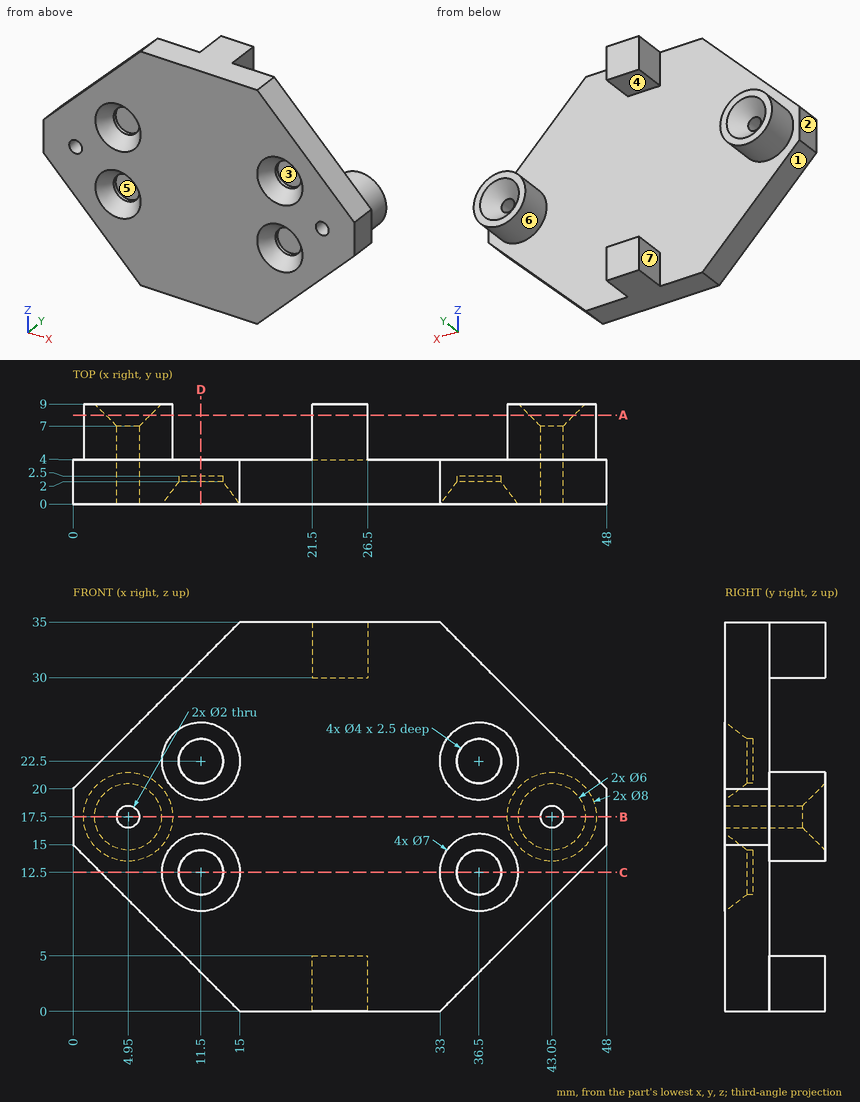
Input: dimensioned drawing with shaded views. Units: mm. Origin: part minimum x, y, z. A direction names the side the tool comes from. Coordinates: 2 decimals unless noted, no trailing zeros. Order: outer loops, then holes, each group sorted by start corner. A loop starts at its lowest first (then second) coordinate and runs counter-clockwise, first axis right, second up. Notation, with made-up numbers: (24.5, -2) -> (73.5, -2) arc R19 cw to (73.5, 19) -> close; hole circle Ø1 at (-2, 87). An arc over 180 degrees is marked (long way). Use CSV: the item, a comma, the result in double quotes.
1) Mould query, pull axis Z, two halves, no side actions, for the marked faces 1, 2, 3 and 4. Classes: +Z half, -Z half, draft (parallel to the pull), parting line (faces both ways), or undercut.
Findings:
face 1,"-Z half"
face 2,"draft"
face 3,"undercut"
face 4,"undercut"
2) Section A-A on y = 8. Output: boundary loops of the cut face in (x, z).
Findings:
outline,"circle Ø8 at (4.95, 17.5); (21.5, 0) -> (26.5, 0) -> (26.5, 5) -> (21.5, 5) -> close; (21.5, 30) -> (26.5, 30) -> (26.5, 35) -> (21.5, 35) -> close; circle Ø8 at (43.05, 17.5); hole circle Ø4 at (4.95, 17.5); hole circle Ø4 at (43.05, 17.5)"
3) Line query: line 1 (Z direction, x = 24, y = 8.25); line 2 (Z direction, x = 36.5, y = 2.3); line 3 (X direction, y = 3.5, z = 17.5). Output: solid intervals per line, ascending.
Findings:
line 1,"z = 0 to 5, 30 to 35"
line 2,"z = 3.5 to 10.5, 14.5 to 20.5, 24.5 to 31.5"
line 3,"x = 0 to 3.95, 5.95 to 42.05, 44.05 to 48"
4) Section D-D on x = 11.5. Output: boundary loops of the cut face in (y, z).
Findings:
outline,"(0, 3.5) -> (4, 3.5) -> (4, 31.5) -> (0, 31.5) -> (0, 26) -> (2, 24.5) -> (2.5, 24.5) -> (2.5, 20.5) -> (2, 20.5) -> (0, 19) -> (0, 16) -> (2, 14.5) -> (2.5, 14.5) -> (2.5, 10.5) -> (2, 10.5) -> (0, 9) -> close"
5) Access query for the marked faces 5, 6 and 7. Directions: +Z, -Z, +X, -X, +Y, -Y. A direction counts if a zero-diameter tool reaches every point of the face in a straight line with its end or side. Return the directions, or none.
Findings:
face 5,"-Y"
face 6,"+Y"
face 7,"+Z, -Z, -X, +Y"
6) Section C-C on z = 12.5. Output: boundary loops of the cut face in (x, y).
Findings:
outline,"(2.5, 0) -> (8, 0) -> (9.5, 2) -> (9.5, 2.5) -> (13.5, 2.5) -> (13.5, 2) -> (15, 0) -> (33, 0) -> (34.5, 2) -> (34.5, 2.5) -> (38.5, 2.5) -> (38.5, 2) -> (40, 0) -> (45.5, 0) -> (45.5, 4) -> (2.5, 4) -> close"
7) Section B-B on z = 17.5. Output: boundary loops of the cut face in (x, y), then the cut area to 3 significant figures.
Findings:
outline,"(0, 0) -> (3.95, 0) -> (3.95, 7) -> (1.95, 9) -> (0.95, 9) -> (0.95, 4) -> (0, 4) -> close; (5.95, 0) -> (42.05, 0) -> (42.05, 7) -> (40.05, 9) -> (39.05, 9) -> (39.05, 4) -> (8.95, 4) -> (8.95, 9) -> (7.95, 9) -> (5.95, 7) -> close; (44.05, 0) -> (48, 0) -> (48, 4) -> (47.05, 4) -> (47.05, 9) -> (46.05, 9) -> (44.05, 7) -> close"
area,"228 mm^2"
8) Pin query (flat end, axial travel): pin 1 Ø3.5 at (x, z) = (11.5, 12.5) entering from -Y; pin 2 Ø4 at (x, z) = (9, 10.5) entering from -Y; pin 3 Ø6.5 at (x, z) = (36.5, 12.5) entering from +Y; pin 4 Ø2.5 at (x, z) = (4.95, 17.5) entering from +Y. Return the tip coordinate at first contact, or that it passes through.
Findings:
pin 1,"stops at y = 2.5"
pin 2,"stops at y = 0"
pin 3,"stops at y = 4"
pin 4,"stops at y = 7.25"
